```python
from build123d import *

# Parameters (mm, degrees)
F0_R     = 32.5
F1_DEPTH = 50
F2_SIZE  = 5
F4_D     = 18


with BuildPart() as f1:
    # F0 (on Front) → F1 (new body)
    with BuildSketch(Plane.XZ):
        Polygon((30, 55), (0, 55), (-30, 55), (-55, 30.6), (-55, -29.4), (-105, -29.4), (-105, -55), (0, -55), (105, -55), (105, -29.4), (55, -29.4), (55, 30.6), align=None)
        Circle(F0_R, mode=Mode.SUBTRACT)
    extrude(amount=-F1_DEPTH)

    # F2
    f2_edges = [f1.edges().sort_by_distance(p)[0] for p in [
        (105, 25, -29.4),
        (-105, 25, -29.4),
    ]]
    chamfer(f2_edges, length=F2_SIZE)

    # F4 (through all)
    with Locations(Plane(origin=(0, 0, -55), x_dir=(1, 0, 0), z_dir=(0, 0, -1))):
        with Locations((-80, -25.4), (80, -25.4)):
            Hole(F4_D / 2)


solid = f1.part
```
Design review of the part built by this model. Coordinates are the model's own, in mm. A direction names the side the tool comes from. Coordinates: 2 decimals unless noted, no trailing zeros. Order: outer loops, then holes, each group sorted by start corner. A loop starts at its lowest first (then second) coordinate and runs counter-clockwise, first axis right, second up. Notation, with made-up numbers: (-35, -35.5) - (17, -35.5) arc R7 ccw to (17, -26.5) - close; hole circle Ø10 at (-36.5, 11.5). An arc over 180 degrees is marked (long way). Answer in a Markdown table with one row per item.
(1) Wall thickness on line 1 along X through (y, z) = (25, -42); line 2 along Y through (x, z) = (-80, -41); line 3 along Z through (x, y) = (0, 16): over which ranges is each line inside the solid? List them lowest first. Write a range as from..to.
Checked values:
| item | result |
|---|---|
| line 1 | -105..-88.99, -71.01..71.01, 88.99..105 |
| line 2 | 0..16.4, 34.4..50 |
| line 3 | -55..-32.5, 32.5..55 |
(2) Clearance check with flat-ended pins moving along their axes: pin 1 (13.5 mm diameter, centred on x = 80, y = 14, fed in from +Z); pin 2 (3 mm diameter, centred on y = 11.5, z = 22, fed in from +X); pin 3 (5 mm diameter, centred on y = 37.5, z = 38, fed in from -X). State where each tip first meets the part, or that it passes through.
Checked values:
| item | result |
|---|---|
| pin 1 | z = -29.4 |
| pin 2 | x = 55 |
| pin 3 | x = -49.98 |
(3) Consider section D-D on y = 6.5. State the section outline as (x, z) points, plus the area to 3 significant figures.
Checked values:
| item | result |
|---|---|
| outline | (-105, -55) - (105, -55) - (105, -34.4) - (100, -29.4) - (55, -29.4) - (55, 30.6) - (30, 55) - (-30, 55) - (-55, 30.6) - (-55, -29.4) - (-100, -29.4) - (-105, -34.4) - close; hole circle Ø65 at (0, 0) |
| area | 10,700 mm^2 |
(4) Consider section B-B on y = 25.4. State the section outline as (x, z) points.
Checked values:
| item | result |
|---|---|
| outline | (-105, -55) - (-89, -55) - (-89, -29.4) - (-100, -29.4) - (-105, -34.4) - close; (-71, -55) - (71, -55) - (71, -29.4) - (55, -29.4) - (55, 30.6) - (30, 55) - (-30, 55) - (-55, 30.6) - (-55, -29.4) - (-71, -29.4) - close; (89, -55) - (105, -55) - (105, -34.4) - (100, -29.4) - (89, -29.4) - close; hole circle Ø65 at (0, 0) |
(5) The part is to be moulded in two halves that separate along X. For faces 4 (the cylindrical face through (71.416, 22.697, -42.021)), 5 (the flat face through (102.5, 24.7, -31.9)), 6 (the flat face through (-42.325, 24.65, 42.971)), say which applies: released by +X, released by -X, zero draft, split by the parting line, or undercut.
Checked values:
| item | result |
|---|---|
| face 4 | undercut |
| face 5 | released by +X |
| face 6 | released by -X |
(6) Consider section C-C on x = 80. State the section outline as (y, z) points, plus the area to 3 significant figures.
Checked values:
| item | result |
|---|---|
| outline | (0, -55) - (16.4, -55) - (16.4, -29.4) - (0, -29.4) - close; (34.4, -55) - (50, -55) - (50, -29.4) - (34.4, -29.4) - close |
| area | 819 mm^2 |
(7) Consider section A-A on z = 0. State the section outline as (x, y) points, plus the area to 3 significant figures.
Checked values:
| item | result |
|---|---|
| outline | (-55, 0) - (-32.5, 0) - (-32.5, 50) - (-55, 50) - close; (32.5, 0) - (55, 0) - (55, 50) - (32.5, 50) - close |
| area | 2,250 mm^2 |
(8) For faces 1 (the flat face through (-55, 25, 1)), 2 (the flat face through (-1, 50, -36)), 3 (the flat face through (73, 19, -29.4)), list the 3-axis set-ups (+Z, -Z, +X, -X, +Y, -Y) from which the entire face can be reached by the end or side of a thin tool; tool diameter is ignored.
Checked values:
| item | result |
|---|---|
| face 1 | +Z, -X, +Y, -Y |
| face 2 | +Z, -Z, +X, -X, +Y |
| face 3 | +Z, +X, +Y, -Y |
